from build123d import *

# Parameters (mm, degrees)
PAD_DEPTH    = 16
PAD001_DEPTH = 4
SKETCH002_R  = 4
POCKET_DEPTH = 16.001
SKETCH003_W  = 16
SKETCH003_H  = 16
PAD002_DEPTH = 4


with BuildPart() as part:
    # Sketch → Pad (new body)
    with BuildSketch(Plane.XZ):
        Polygon((0, 0), (0, 100), (16, 100), (16, 16), (50, 16), (50, -100), (34, -100), (34, 0), align=None)
    extrude(amount=PAD_DEPTH)

    # Sketch001 (on Face10 of Pad) → Pad001 (join)
    with BuildSketch(Plane.XZ.offset(16)):
        Polygon((0, 0), (50, 0), (50, 16), (16, 50), (0, 50), align=None)
        Polygon((16, 16), (40, 16), (16, 40), align=None, mode=Mode.SUBTRACT)
    extrude(amount=PAD001_DEPTH)

    # Sketch002 (on Face14 of Pad001) → Pocket (cut, through all)
    with BuildSketch(Plane(origin=(16, 0, 0), x_dir=(0, 0, 1), z_dir=(1, 0, 0))):
        with Locations((30, 8)):
            Circle(SKETCH002_R)
    extrude(amount=-POCKET_DEPTH, mode=Mode.SUBTRACT)

    # Sketch003 (on Face2 of Pocket) → Pad002 (join)
    with BuildSketch(Plane(origin=(0, 0, 0), x_dir=(0, 0, -1), z_dir=(-1, 0, 0))):
        with Locations((-92, 8)):
            Rectangle(SKETCH003_W, SKETCH003_H)
    extrude(amount=PAD002_DEPTH)


solid = part.part
Verification items for the finished model (mm, model axes). A direction names the side the tool comes from. Give positions to 0.01 mm unless a question says otherwise; leave off trailing zeros. Loops run counter-clockwise (first coordinate to the right, second up) from the corner with the lowest first, then second, coordinate; pieces in that order, holes last. Notation, with made-up numbers: (-21, -33) - (19, -33) arc R28 cw to (19, -12) - close; hole circle Ø2 at (64, 74). An arc over 180 degrees is marked (long way). Write each question's results on one line, items separated by ' | '.
1) Sectioned sample at C-C on y = -8. Record the boundary of the cut face in (x, z).
Solution:
outline: (-4, 84) - (0, 84) - (0, 34) - (16, 34) - (16, 100) - (-4, 100) - close; (0, 0) - (34, 0) - (34, -100) - (50, -100) - (50, 16) - (16, 16) - (16, 26) - (0, 26) - close
2) Depth check by flat-ended pin: P1, Ø6, axis at x = 20, y = -4, coming from the +Z side; P2, Ø16, axis at x = 8, z = 72.5, coming from the -Y side; P3, Ø8, axis at x = 17, y = -17, coming from the -Z side. Enter the tip coordinate at first touch or a pass-through.
Solution:
P1: z = 16 | P2: y = -16 | P3: z = 0
3) Material ranges on L1, parallel to Z at x = 3.5, y = -8; L2, parallel to Z at x = 8, y = -15.75; L3, parallel to X at y = -10.75, z = -32, recorded low to high. Write a range as from..to.
Solution:
L1: 0..26, 34..100 | L2: 0..100 | L3: 34..50
4) Sectioned sample at A-A on z = 30. Record the boundary of the cut face in (x, y).
Solution:
outline: (0, -20) - (16, -20) - (16, -12) - (0, -12) - close; (0, -4) - (16, -4) - (16, 0) - (0, 0) - close; (26, -20) - (36, -20) - (36, -16) - (26, -16) - close
5) Sectioned sample at B-B on x = 21.5. Record the boundary of the cut face in (y, z), plus the area to 3 significant figures.
Solution:
outline: (-20, 0) - (0, 0) - (0, 16) - (-20, 16) - close; (-20, 34.5) - (-16, 34.5) - (-16, 44.5) - (-20, 44.5) - close | area: 360 mm2
6) Mould release check, pull along Z, two halves, no side actions. Record for faces 6 (the flat face through (8, -18, 50)), 7 (the cylindrical face through (8.1, -5.6, 26.8)), 8 (the flat face through (-2, -8, 84)): pulls with the +Z half, pulls with the -Z half, needs draft (parallel to the pull), parting line crosses it, or undercut.
Solution:
face 6: pulls with the +Z half | face 7: undercut | face 8: pulls with the -Z half
7) Tool access check on faces 1 (the flat face through (33, -10, 16)), 2 (the flat face through (30, -16, 31)), 3 (the flat face through (42, -16, -49)), 4 (the flat face through (8, -16, 75)), 5 (the flat face through (0, -10, 43)). Record the directions out of +Z, -Z, +X, -X, +Y, -Y that give a thin tool (end or side, any length) a straight path to the whole face; none if there is none.
Solution:
face 1: +Y | face 2: +Z, +X, +Y | face 3: -Z, +X, -X, -Y | face 4: +Z, +X, -X, -Y | face 5: -Z, -X, +Y, -Y
8) Sectioned sample at D-D on x = 11. Record the boundary of the cut face in (y, z).
Solution:
outline: (-20, 0) - (0, 0) - (0, 100) - (-16, 100) - (-16, 50) - (-20, 50) - close; hole circle Ø8 at (-8, 30)
